The listing builds one solid part. Answer for the finished solid, in the listing's coordinates (mm). A direction names the side the tool comes from. Give positions to 0.01 mm unless a question says otherwise; leave off trailing zeros. Loops run counter-clockwise (first coordinate to the right, second up) from the corner with the lowest first, then second, coordinate; pieces in that order, holes last. Notation, with made-up numbers: M 8,-38 L 18,-38 A25 cw 18,-19 Z; hole C 50.5,56 d11. An arc over 180 degrees is marked long. One line per item, written item: value. Start each with the question number.
Q1. A cutting plane is placed at C-C, the plane z = -2. Determine the outline of the cut face in (x, y).
Q2. A cutting plane is placed at B-B, the plane y = 2.9. Determine the outline of the cut face in (x, z), and give its area (3 significant figures).
Q3. The mould has two halves that part along X. Classify faces 1 (the flat face through (25, 2, 0)), 2 (the flat face through (0, 2, 20)), 3 (the cylindrical face through (-0.61, 0.99, -10.36)): +X half, -X half, draft (parallel to the pull), parting line (faces both ways), or undercut.
Q4. For faces 4 (the flat face through (3, 2, -5)), 5 (the cylindrical face through (15.502, 1.972, 1.015)), determine the directions among +Z, -Z, +X, -X, +Y, -Y from which every point of the face is accessible in a straight line to the end or side of a thin tool.
Q5. A cutting plane is placed at A-A, the plane x = -17.5. Determine the outline of the cut face in (y, z).
Q6. A flat-ended cylindrical pin translates along its axis: pin 1 (3 mm diameter, centred on x = -17.5, z = 1.1, fed in from +Y). Find the tip coordinate at first contact, or state that the pin passes through.
Q7. Consider L1, parallel to Z at x = 17.5, y = 2.2; L2, parallel to Z at x = 17, y = 3.8; L3, parallel to X at y = 2.3, z = -6.5. Determine where each line is inside the solid, lowest interval first.
from build123d import *

# Parameters (mm, degrees)
SKETCH1_R           = 2
SKETCH1_R_2         = 14
SKETCH1_R_3         = 4.5
SKETCH1_R_4         = 3
BOSS_EXTRUDE2_DEPTH = 4
SKETCH1_14_R        = 3
CUT_EXTRUDE2_DEPTH  = 5
SKETCH1_15_R        = 4.5
CUT_EXTRUDE3_DEPTH  = 2


with BuildPart() as part:
    # Sketch1 → Boss-Extrude2 (new body)
    with BuildSketch(Plane(origin=(0, 0, 0), x_dir=(1, 0, 0), z_dir=(0, 1, 0))):
        with BuildLine():
            Line((21.446973136, 20), (-21.446973136, 20))
            ThreePointArc((-21.446973136, 20), (-23.935145745, 18.935145745), (-25, 16.446973136))
            Line((-25, 16.446973136), (-25, 16.276952121))
            Line((-25, 16.276952121), (-25, -16.276952121))
            Line((-25, -16.276952121), (-25, -16.446973136))
            ThreePointArc((-25, -16.446973136), (-23.935145745, -18.935145745), (-21.446973136, -20))
            Line((-21.446973136, -20), (21.446973136, -20))
            ThreePointArc((21.446973136, -20), (23.935145745, -18.935145745), (25, -16.446973136))
            Line((25, -16.446973136), (25, -16.276952121))
            Line((25, -16.276952121), (25, 16.276952121))
            Line((25, 16.276952121), (25, 16.446973136))
            ThreePointArc((25, 16.446973136), (23.935145745, 18.935145745), (21.446973136, 20))
        make_face()
        with Locations((-17.5, -1.102660735)):
            Circle(SKETCH1_R, mode=Mode.SUBTRACT)
        with Locations((17.5, -1.102660735)):
            Circle(SKETCH1_R, mode=Mode.SUBTRACT)
        Circle(SKETCH1_R_2, mode=Mode.SUBTRACT)
        Circle(SKETCH1_R_2)
        with Locations((-0.021660512, 5.8998827)):
            Circle(SKETCH1_R_3, mode=Mode.SUBTRACT)
        with Locations((-0.021660512, 5.8998827)):
            Circle(SKETCH1_R_3)
        with Locations((-0.021660512, 5.8998827)):
            Circle(SKETCH1_R_4, mode=Mode.SUBTRACT)
        with Locations((-0.021660512, 5.8998827)):
            Circle(SKETCH1_R_4)
    extrude(amount=BOSS_EXTRUDE2_DEPTH)

    # Sketch1_14 → Cut-Extrude2 (cut, through all)
    with BuildSketch(Plane(origin=(0, 0, 0), x_dir=(1, 0, 0), z_dir=(0, 1, 0))):
        with Locations((-0.021660512, 5.8998827)):
            Circle(SKETCH1_14_R)
    extrude(amount=CUT_EXTRUDE2_DEPTH, mode=Mode.SUBTRACT)

    # Sketch1_15 → Cut-Extrude3 (cut)
    with BuildSketch(Plane(origin=(0, 0, 0), x_dir=(1, 0, 0), z_dir=(0, 1, 0))):
        with Locations((-0.021660512, 5.8998827)):
            Circle(SKETCH1_15_R)
    extrude(amount=CUT_EXTRUDE3_DEPTH, mode=Mode.SUBTRACT)


solid = part.part
Answer block:
1. outline: M -25,0 L -2.27,0 L -2.27,2 L 2.22,2 L 2.22,0 L 25,0 L 25,4 L -25,4 Z
2. outline: M -25,-16.45 A3.64 ccw -21.45,-20 L 21.45,-20 A3.64 ccw 25,-16.45 L 25,16.45 A3.64 ccw 21.45,20 L -21.45,20 A3.64 ccw -25,16.45 Z; hole C -17.5,1.1 d4; hole C -0.02,-5.9 d6; hole C 17.5,1.1 d4
2. area: 1,940 mm^2
3. face 1: +X half
3. face 2: draft
3. face 3: undercut
4. face 4: -Y
4. face 5: +Y, -Y
5. outline: M 0,-20 L 4,-20 L 4,-0.9 L 0,-0.9 Z; M 0,3.1 L 4,3.1 L 4,20 L 0,20 Z
6. pin 1: through
7. L1: -20 to -0.9, 3.1 to 20
7. L2: -20 to -0.83, 3.04 to 20
7. L3: -25 to -2.96, 2.92 to 25
